Could you check a few things on this model? Use its own coordinates, in mm. A direction names the side the tool comes from. Round coordinates to 2 decimals unless told otherwise and drop trailing zeros. Answer as CSV lines item,"result". Start each with the question number.
1) Suppose I cut it at A-A, the plane y = 14.5. Count the separate pieces of the cut face and the enclosed holes in it, then the cut area to 3 significant figures.
2) Which directions (+Z, -Z, +X, -X, +Y, -Y) give clear straight access to the entire face, cutting with the end or side of a thin tool? Please do faces 1 (the face through (2.5, 5, -10)), 2 (the face through (12, -4, -12)), 3 (the face through (17.282, -1.172, -8.923)).
3) Please list where these lines run through material, in increasing order: line 1 along X through (y, z) = (8.5, 10); line 2 along Z through (x, y) = (11.5, 0); line 3 along X through (y, z) = (-12.5, 9).
4) We'd pull the mould along Y, two halves only. Please class faces 4 (the face through (7.8, 0, 0)), 5 (the face through (9, 4, -12)), 6 (the face through (5.5, -1.5, -11.4)), 7 (the face through (14, -6, 0)): pulls with the +Y half, pulls with the -Y half, needs draft (parallel to the pull), parting line crosses it, or undercut.
5) I'm going to push flat-ended pins straight in: pin 1 Ø4 at (x, z) = (13, -13) entering from +Y; pin 2 Ø2 at (x, y) = (7.5, -11.5) entering from -Z; pin 3 Ø1.5 at (x, y) = (14.5, -1.5) entering from -Z. Where does each tip first touch, or does it pass through?
```python
from build123d import *


with BuildPart() as part:
    # Esquisse1 → Révolution1 (revolve)
    with BuildSketch(Plane.XY):
        with BuildLine():
            Line((0, 0), (0, 8.5))
            Line((0, 8.5), (2.5, 11))
            Line((2.5, 11), (2.5, 15))
            Line((2.5, 15), (3.5, 16))
            Line((3.5, 16), (4, 16))
            Line((4, 16), (4, 12.826466888))
            Line((4, 12.826466888), (4, 11.5))
            Line((4, 11.5), (7, 11.5))
            Line((7, 11.5), (7, 17.18964629))
            Line((7, 17.18964629), (7.3, 17.48964629))
            Line((7.3, 17.48964629), (8.7, 17.48964629))
            Line((8.7, 17.48964629), (9, 17.18964629))
            Line((9, 17.18964629), (9, 12))
            Line((9, 12), (12, 12))
            Line((12, 12), (12, 17.18964629))
            Line((12, 17.18964629), (12.3, 17.48964629))
            Line((12.3, 17.48964629), (12.7, 17.48964629))
            Line((12.7, 17.48964629), (13, 17.18964629))
            Line((13, 17.18964629), (13, 11))
            ThreePointArc((13, 11), (13.585786438, 9.585786438), (15, 9))
            Line((15, 9), (19.5, 9))
            Line((19.5, 9), (19.8, 8.7))
            Line((19.8, 8.7), (19.8, 6))
            Line((19.8, 6), (7.8, 6))
            Line((7.8, 6), (7.8, 0))
            Line((7.8, 0), (0, 0))
        make_face()
    revolve(axis=Axis((7.8, 0, 0), (-1, 0, 0)))


solid = part.part
```
Filled sheet:
1,separate pieces,"3"
1,enclosed holes,"0"
1,area,"75.6 mm²"
2,face 1,"-X"
2,face 2,"none"
2,face 3,"+X"
3,line 1,"2.5 to 4, 7 to 9, 12 to 13"
3,line 2,"-12 to -6, 6 to 12"
3,line 3,"2.9 to 4, 7 to 9, 12 to 13"
4,face 4,"undercut"
4,face 5,"needs draft"
4,face 6,"parting line crosses it"
4,face 7,"undercut"
5,pin 1,"y = 13.58"
5,pin 2,"z = -13.99"
5,pin 3,"z = -9.33"
